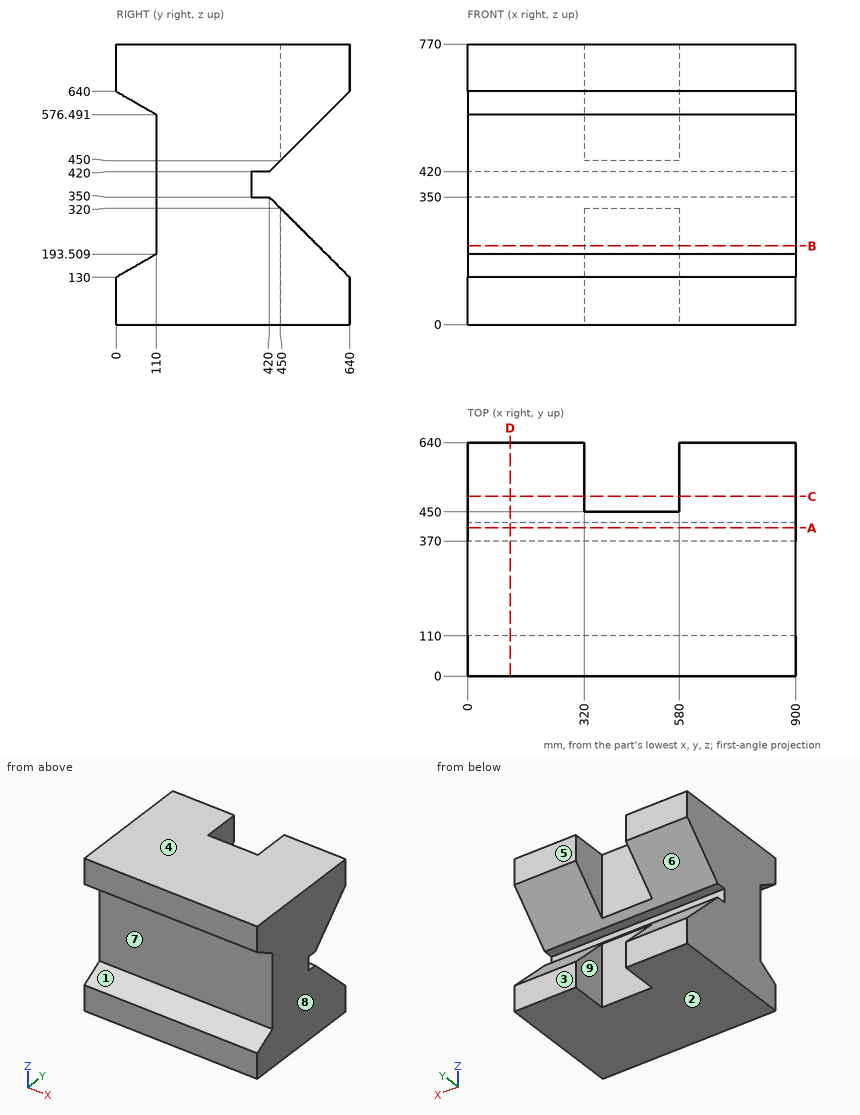
Source: three-view drawing plus pictorial views. Frame: mm from the lowest corner of the part. A direction names the side the tool comes from. Give positions to 0.01 mm unless a question says otherwise; leave off trailing zeros. Write each loop counter-clockwise with the first axis right and the second up, starting at its lowest first coordinate (ties: lowest second). Pieces come first, ordered by that corner, then holes.
(1) Cut plane A-A, the plane y = 406. Return loops of the section in (x, z).
(2) Cut plane C-C, the plane y = 493. Return loops of the section in (x, z).
(3) Cut plane B-B, the plane z = 216.5. Return loops of the section in (x, y), then the cut area to 3 significant figures.
(4) First-contact query: P1, Ø8, axis at y = 523.5, z = 512.5, coming from the -X side. Flat tip, straight axial feed; report the tip coordinate or a pass-through.
(5) Ray query, line 1 (Y direction, x = 578, z = 514); line 2 (Z direction, x = 791, y = 505); line 3 (Y direction, x = 781, z = 387). Return the intervals inside material, ascending.
(6) Mould query, pull axis Z, two halves, no side actions, for the marked faces 1, 2, 3 and 4. Classes: released by +Z, released by -Z, zero draft, split by the parting line, or undercut.
(7) Cut plane D-D, the plane x = 116.5. Return loops of the section in (y, z).
(8) Access query for the marked faces 5, 6, 7, 8 and 9. Directions: +Z, -Z, +X, -X, +Y, -Y. A direction counts if a zero-diameter tool reaches every point of the face in a straight line with its end or side. Return the directions, or none.
Values follow:
1. outline: (0, 0) - (900, 0) - (900, 350) - (0, 350) - close; (0, 420) - (900, 420) - (900, 770) - (0, 770) - close
2. outline: (0, 0) - (320, 0) - (320, 277) - (0, 277) - close; (0, 493) - (320, 493) - (320, 770) - (0, 770) - close; (580, 0) - (900, 0) - (900, 277) - (580, 277) - close; (580, 493) - (900, 493) - (900, 770) - (580, 770) - close
3. outline: (0, 110) - (900, 110) - (900, 553.5) - (580, 553.5) - (580, 450) - (320, 450) - (320, 553.5) - (0, 553.5) - close
3. area: 372,000 mm2
4. P1: passes through
5. line 1: y = 110 to 450
5. line 2: z = 0 to 265, 505 to 770
5. line 3: y = 110 to 370
6. face 1: undercut
6. face 2: released by -Z
6. face 3: zero draft
6. face 4: released by +Z
7. outline: (0, 0) - (640, 0) - (640, 130) - (420, 350) - (370, 350) - (370, 420) - (420, 420) - (640, 640) - (640, 770) - (0, 770) - (0, 640) - (110, 576.49) - (110, 193.51) - (0, 130) - close
8. face 5: +Z, -Z, +X, -X, +Y
8. face 6: +X, -X, +Y
8. face 7: +X, -X, -Y
8. face 8: +Z, -Z, +X, +Y, -Y
8. face 9: +Z, -Z, +Y
